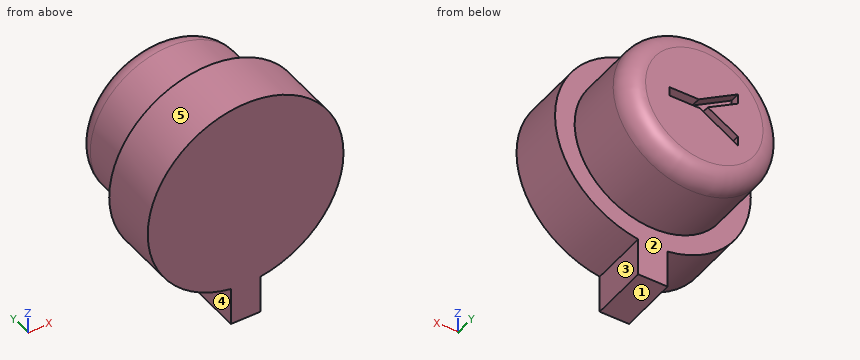
Autodesk Inventor part; units mm, degrees
ref_plane "YZ Plane" through (0, 0, 0) normal (1, 0, 0) x (0, 1, 0)
ref_plane "XZ Plane" through (0, 0, 0) normal (0, 1, 0) x (-1, 0, 0)
ref_plane "XY Plane" through (0, 0, 0) normal (0, 0, 1) x (1, 0, 0)
sketch "Skizze1" plane through (0, 0, 0) normal (1, 0, 0) x (0, 1, 0)
  line L0 (4, 0) -> (4, 3)
  arc A0 (4, 3) -> (3, 4) centre (3, 3) ccw
  line L1 (3, 4) -> (0, 4)
  line L2 (0, 4) -> (0, 5)
  line L3 (0, 5) -> (-3, 5)
  line L4 (-3, 5) -> (-3, 2)
  line L5 (0, 0) -> (4, 0)
  line L6 (-3, 2) -> (-3, 0)
  line L7 (-3, 0) -> (0, 0)
  point P0 (0, 2)
  dimension "d0" = 2
  dimension "d1" = 4
  dimension "d2" = 3
  dimension "d3" = 5
  dimension "d4" = 3
  dimension "d5" = 1
  dimension "d6" = 1
revolve "Umdrehung1" add sketch "Skizze1" angle 360 about axis through (0, 0, 0) along (0, 1, 0)
sketch "Skizze2" plane through (0, 4, 0) normal (0, 1, 0) x (1, 0, 0)
  line L0 (-1.7168, -1.418) -> (-1.7168, 1.5147) construction
  line L1 (-1.7168, 1.5147) -> (1.7832, 1.5147) construction
  line L2 (1.7832, 1.5147) -> (1.7832, -1.418) construction
  line L3 (1.7832, -1.418) -> (-1.7168, -1.418) construction
  line L4 (-1.7168, 1.3871) -> (0.2346, 0.2044)
  line L5 (0.2346, 0.2044) -> (1.7832, 0.2044)
  line L6 (1.7832, 0.2044) -> (1.7832, -0.2608)
  line L7 (1.7832, -0.2608) -> (0.2828, -0.2608)
  line L8 (0.2828, -0.2608) -> (-1.7168, -1.4435)
  line L9 (-1.7168, -1.4435) -> (-1.7168, -0.9273)
  line L10 (-1.7168, -0.9273) -> (-0.1767, -0.0254)
  line L11 (-0.1767, -0.0254) -> (-1.7168, 0.8936)
  line L12 (-1.7168, 0.8936) -> (-1.7168, 1.3871)
  point P0 (0, 0)
extrude "Extrusion1" cut sketch "Skizze2" against normal blind 0.5
sketch "Skizze4" plane through (0, -3, 0) normal (0, -1, 0) x (1, 0, 0)
  line L0 (0.75, -4.8836) -> (-0.75, -4.8836)
  line L1 (-0.75, -4.8836) -> (-0.75, -6.8836)
  line L2 (-0.75, -6.8836) -> (0.75, -6.8836)
  line L3 (0.75, -6.8836) -> (0.75, -4.8836)
  point P0 (0, 0)
  dimension "d15" = 1.5
  dimension "d16" = 2
  dimension "d17" = 0.75
extrude "Extrusion3" add sketch "Skizze4" against normal blind 3
properties part number "ButtonY_neu"
For this review, take the finished solid that the model builds, in its own axes (mm). Face numbers are marked on the shaded views. A direction names the side the tool comes from. Coordinates: 2 decimals unless noted, no trailing zeros. Loops run counter-clockwise (first coordinate to the right, second up) from the corner with the lowest first, then second, coordinate; pieces in that order, holes last. Notation, with made-up numbers: (-23, -39.75) - (-2, -39.75) arc R31 ccw to (-2, -0.75) - close; hole circle Ø2 at (61, 30.25). An arc over 180 degrees is marked (long way). Return JSON: item names as keys, results as strings.
Item 1: For the marked faces 1, 2, 3, 4 and 5, list the 3-axis set-ups (+Z, -Z, +X, -X, +Y, -Y) from which the entire face can be reached by the end or side of a thin tool; tool diameter is ignored.
Determined:
{"face 1": "-Z, +X, -X, +Y, -Y", "face 2": "+Y", "face 3": "-Z, +X, +Y, -Y", "face 4": "-Z, -X, +Y, -Y", "face 5": "+Y, -Y"}
Item 2: Take a section at D-D (y = 0.25). Give the boundary of the cut face in (x, z), then the cut area to 3 significant figures.
Determined:
{"outline": "circle Ø8 at (0, 0)", "area": "50.3 mm2"}
Item 3: Take a section at A-A (x = 0). Give the boundary of the cut face in (y, z).
Determined:
{"outline": "(-3, -6.88) - (0, -6.88) - (0, -4) - (3, -4) arc R1 ccw to (4, -3) - (4, -0.35) - (3.5, -0.35) - (3.5, 0.43) - (4, 0.43) - (4, 3) arc R1 ccw to (3, 4) - (0, 4) - (0, 5) - (-3, 5) - close"}
Item 4: Take a section at B-B (y = -2). Give the boundary of the cut face in (x, z).
Determined:
{"outline": "(-0.75, -6.88) - (0.75, -6.88) - (0.75, -4.94) arc R5 ccw (long way) to (-0.75, -4.94) - close"}
Item 5: Take a section at C-C (z = 4.25). Give the boundary of the cut face in (x, y), then the cut area to 3 significant figures.
Determined:
{"outline": "(-2.63, -3) - (2.63, -3) - (2.63, 0) - (-2.63, 0) - close", "area": "15.8 mm2"}
Item 6: For line 1 (X direction, y = -0.75, z = 3); line 2 (Y direction, x = -0.25, z = -5); line 3 (X direction, y = -1, z = 4), list the stretches that pass through material, from the lowest coordinate up.
Determined:
{"line 1": "x = -4 to 4", "line 2": "y = -3 to 0", "line 3": "x = -3 to 3"}
Item 7: Insertion check: pin 1 (4 mm diameter, centred on y = 1.5, z = -2, fed in from -X); pin 2 (0.5 mm diameter, centred on y = 4, z = -1.5, fed in from +X); pin 3 (1.6 mm diameter, centred on y = -2, z = -6.5, fed in from +X). Each pin has a flat end and moves straight along its axis. Give the tip position at first contact, or say it passes through.
Determined:
{"pin 1": "stops at x = -4.95", "pin 2": "stops at x = 3.36", "pin 3": "stops at x = 0.75"}
